Part model, mm, in its own coordinate system. A direction names the side the tool comes from. Round coordinates to 2 decimals unless told otherwise and drop trailing zeros. Write each loop counter-clockwise with the first axis right and the second up, starting at its lowest first coordinate (ties: lowest second). Pieces come first, ordered by that corner, then holes. Notation, with made-up numbers: M 5,42 L 11,42 A13 ccw 11,59 Z; hole C 65,-14.75 d8. An arc over 180 degrees is marked long. Answer as a JSON object with one key per item and string values. Group by question number.
1. Drop flat-ended pins along their axis: pin 1 (6 mm diameter, centred on x = 32, y = -14, fed in from -Z); pin 2 (14.5 mm diameter, centred on x = 6.5, y = -9, fed in from +Z); pin 3 (2 mm diameter, centred on x = -4, y = -6.5, fed in from +Z); pin 4 (22.5 mm diameter, centred on y = -10, z = -27, fed in from -X). Give the stop position or say it passes through.
2. Two-plate mould, pull along Y, no slides. Class faces 1 (the face through (23, 10, -59)), 2 (the face through (30.86, -9.86, 6.52)), 3 (the face through (22.96, -0.79, -58.55)): +Y half, -Y half, draft (parallel to the pull), parting line (faces both ways), or undercut.
3. Band-saw the part on D-D, the plane y = -16.5. Write the cut outline in (x, z).
4. Drill centre lines: line 1 (Z direction, x = 0, y = -8); line 2 (X direction, y = -1, z = -41.5); line 3 (Z direction, x = 38, y = -19). Where is each one in solid material? Low to high. Write a range as from..to.
5. Band-saw the part on C-C, the plane x = 24. Write the cut outline in (y, z), plus the area to 3 significant figures.
6. Band-saw the part on A-A, the plane y = -10. Write the cut outline in (x, z).
7. Which spindle directions (+Z, -Z, +X, -X, +Y, -Y) get a long thin tool onto all of the face, cutting with end or side? Do faces 4 (the face through (32, -10, 0)), 5 (the face through (9, -10, 12)), 6 (the face through (23, 5, 7)). Say none if no direction does.
8. Band-saw the part on B-B, the plane z = -107. Write the cut outline in (x, y).
from build123d import *

# Parameters (mm, degrees)
F0_R          = 8
F0_R_2        = 9
F1_DEPTH      = 20
F2_W          = 6
F2_H          = 144
F3_DEPTH      = 10
F3_DEPTH_BACK = 30
F4_SIZE       = 10
F5_T1_DEPTH   = 20
F6_R          = 12.5
F7_DEPTH      = 6


# Not quite as in the source:
# - a fillet or chamfer that OpenCascade refuses, or shapes differently, is made with other operations: its cross-section is extruded or revolved along the edge and cut away or added


with BuildPart() as f1:
    # F0 (on Front) → F1 (new body)
    with BuildSketch(Plane.XZ):
        with BuildLine():
            ThreePointArc((0, 12), (-8.4852813742, -8.4852813742), (12, 0))
            ThreePointArc((12, 0), (8.4852813742, 8.4852813742), (0, 12))
        make_face()
        Circle(F0_R, mode=Mode.SUBTRACT)
        with BuildLine():
            ThreePointArc((0, 12), (8.4852813742, 8.4852813742), (12, 0))
            Line((12, 0), (38, 0))
            ThreePointArc((38, 0), (29.5147186258, 3.5147186258), (26, 12))
            Line((26, 12), (0, 12))
        make_face()
        with BuildLine():
            ThreePointArc((26, 12), (29.5147186258, 3.5147186258), (38, 0))
            ThreePointArc((38, 0), (46.4852813742, 3.5147186258), (50, 12))
            ThreePointArc((50, 12), (38, 24), (26, 12))
        make_face()
        with Locations((38, 12)):
            Circle(F0_R_2, mode=Mode.SUBTRACT)
    extrude(amount=F1_DEPTH)

    # F2 (on face) → F3 (join, two sides)
    with BuildSketch(Plane.XZ.offset(20)) as f3_sk:
        with Locations((23, -60)):
            Rectangle(F2_W, F2_H)
    extrude(amount=F3_DEPTH)
    extrude(f3_sk.sketch, amount=-F3_DEPTH_BACK)

    # F4
    f4_edges = [f1.edges().sort_by_distance(p)[0] for p in [
        (23, -30, 12),
        (23, 10, 12),
        (23, -30, -132),
        (23, 10, -132),
    ]]
    chamfer(f4_edges, length=F4_SIZE)

    # F5: fillet of radius 10 on 2 edges, made by hand

    # F5_s2 → F5_t1 (join)
    with BuildSketch(Plane.XZ):
        with BuildLine():
            ThreePointArc((18.4040820577, 12), (23.6264117364, 13.4719713458), (27.311317486, 17.4545454545))
            ThreePointArc((27.311317486, 17.4545454545), (26.3324340549, 14.8049785946), (26, 12))
            Line((26, 12), (18.4040820577, 12))
        make_face()
        with BuildLine():
            ThreePointArc((20, -9.7979589711), (17.7459666924, -3.4734036508), (12, 0))
            Line((12, 0), (20, 0))
            Line((20, 0), (20, -9.7979589711))
        make_face()
    extrude(amount=F5_T1_DEPTH)

    # F6 (on face) → F7 (cut, through all)
    with BuildSketch(Plane(origin=(20, 0, 0), x_dir=(0, -1, 0), z_dir=(-1, 0, 0))):
        with Locations((10, -107)):
            Circle(F6_R)
        with Locations((10, -67)):
            Circle(F6_R)
        with Locations((10, -27)):
            Circle(F6_R)
    extrude(amount=-F7_DEPTH, mode=Mode.SUBTRACT)


solid = f1.part
Worked answers:
{
 "1": {"pin 1": "stops at z = 0", "pin 2": "stops at z = 12", "pin 3": "stops at z = 11.62", "pin 4": "passes through"},
 "2": {"face 1": "+Y half", "face 2": "draft", "face 3": "undercut"},
 "3": {"outline": "M 0,12 A12 ccw long 12,0 A10 cw 20,-9.8 L 20,-16.32 L 26,-16.32 L 26,0 L 38,0 A12 ccw long 27.31,17.45 A10 cw 18.4,12 Z; M 20,-132 L 26,-132 L 26,-117.68 L 20,-117.68 Z; M 20,-96.32 L 26,-96.32 L 26,-77.68 L 20,-77.68 Z; M 20,-56.32 L 26,-56.32 L 26,-37.68 L 20,-37.68 Z; hole C 0,0 d16; hole C 38,12 d18"},
 "4": {"line 1": "z = -12..-8, 8..12", "line 2": "x = 20..26", "line 3": "z = 0..3, 21..24"},
 "5": {"outline": "M -30,-122 L -20,-132 L 0,-132 L 10,-122 L 10,2 L 0,12 L 0,13.71 L -20,13.71 L -20,12 L -30,2 Z; hole C -10,-107 d25; hole C -10,-67 d25; hole C -10,-27 d25", "area": "4,120 mm^2"},
 "6": {"outline": "M 0,12 A12 ccw long 12,0 A10 cw 20,-9.8 L 20,-14.5 L 26,-14.5 L 26,0 L 38,0 A12 ccw long 27.31,17.45 A10 cw 18.4,12 Z; M 20,-132 L 26,-132 L 26,-119.5 L 20,-119.5 Z; M 20,-94.5 L 26,-94.5 L 26,-79.5 L 20,-79.5 Z; M 20,-54.5 L 26,-54.5 L 26,-39.5 L 20,-39.5 Z; hole C 0,0 d16; hole C 38,12 d18"},
 "7": {"face 4": "-Z, +X, +Y, -Y", "face 5": "+Z, -X, +Y, -Y", "face 6": "+Z, +X, -X, +Y"},
 "8": {"outline": "M 20,-30 L 26,-30 L 26,-22.5 L 20,-22.5 Z; M 20,2.5 L 26,2.5 L 26,10 L 20,10 Z"}
}
